Could you check a few things on this model? Use its own coordinates, in mm. A direction names the side the tool comes from. Give positions to 0.01 mm unless a question says otherwise; leave off trailing zeros. Loops run counter-clockwise (first coordinate to the right, second up) from the corner with the lowest first, then second, coordinate; pieces in that order, holes last. Notation, with made-up numbers: M -5,-35 L 17,-35 A20 cw 17,-9 Z; hole C 36,-36.5 d8. An arc over 180 degrees is marked long. Use CSV: the item, a comma, the result in double quotes.
```python
from build123d import *

# Parameters (mm, degrees)
BOSS_EXTRUDE1_DEPTH = 50
SKETCH2_W           = 7
SKETCH2_H           = 8
BOSS_EXTRUDE2_DEPTH = 50
SKETCH2_3_W         = 7
SKETCH2_3_H         = 8
BOSS_EXTRUDE3_DEPTH = 18
SKETCH3_W           = 10
SKETCH3_H           = 63
SKETCH3_W_2         = 7
SKETCH3_H_2         = 8
BOSS_EXTRUDE4_DEPTH = 82
FILLET1_R           = 5
SKETCH4_W           = 49
SKETCH4_H           = 29.5
CUT_EXTRUDE1_DEPTH  = 63
SKETCH5_W           = 29.5
SKETCH5_H           = 11
BOSS_EXTRUDE5_DEPTH = 49
CUT_EXTRUDE2_DEPTH  = 29.5
SKETCH6_R           = 1.75
CUT_EXTRUDE3_DEPTH  = 5
SKETCH6_6_R         = 0.75
CUT_EXTRUDE4_DEPTH  = 15
SKETCH8_W           = 18
SKETCH8_H           = 9.5
CUT_EXTRUDE5_DEPTH  = 40
SKETCH9_W           = 7
SKETCH9_H           = 9.5
CUT_EXTRUDE6_DEPTH  = 45
SKETCH10_W          = 10
SKETCH10_H          = 10
CUT_EXTRUDE7_DEPTH  = 29.5
SKETCH11_W          = 13
SKETCH11_H          = 48
SKETCH11_H_2        = 7
CUT_EXTRUDE8_DEPTH  = 124.13610356
SKETCH12_W          = 8
SKETCH12_H          = 10
CUT_EXTRUDE9_DEPTH  = 114.279521539
SKETCH13_W          = 10
SKETCH13_H          = 6
CUT_EXTRUDE10_DEPTH = 14
SKETCH15_W          = 14
SKETCH15_H          = 6
CUT_EXTRUDE11_DEPTH = 128.218316291
FILLET2_R           = 3
SKETCH17_W          = 49
SKETCH17_H          = 62
BOSS_EXTRUDE6_DEPTH = 46.5
CUT_EXTRUDE12_START = -30
SKETCH18_W          = 45
SKETCH18_H          = 63
CUT_EXTRUDE12_DEPTH = 30
SKETCH19_W          = 45
SKETCH19_H          = 4
SKETCH19_H_2        = 27.35
BOSS_EXTRUDE7_DEPTH = 30
BOSS_EXTRUDE8_DEPTH = 3
SKETCH24_W          = 14
SKETCH24_H          = 10
CUT_EXTRUDE15_DEPTH = 112.778799421
SKETCH26_W          = 42
SKETCH26_H          = 31.65
CUT_EXTRUDE16_DEPTH = 8
SKETCH27_W          = 42
SKETCH27_H          = 38
CUT_EXTRUDE17_DEPTH = 7
SKETCH28_W          = 42
SKETCH28_H          = 38
CUT_EXTRUDE18_DEPTH = 7
SKETCH29_W          = 38
SKETCH29_H          = 45.65
CUT_EXTRUDE19_DEPTH = 7
SKETCH30_W          = 46.5
SKETCH30_H          = 6
CUT_EXTRUDE20_DEPTH = 131.599578866
CUT_EXTRUDE21_DEPTH = 127.610623567
SKETCH32_3_R        = 0.9
SKETCH32_3_R_2      = 0.75
CUT_EXTRUDE22_DEPTH = 6


with BuildPart() as part:
    # Sketch1 → Boss-Extrude1 (new body)
    with BuildSketch(Plane.XY):
        with BuildLine():
            Line((-2.25, -8), (-4.25, -8))
            ThreePointArc((-4.25, -8), (-3.25, -8.5), (-2.25, -8))
        make_face()
        Polygon((10, -25.5), (10, 0), (0, 0), (-18, 0), (-18, -8), (0, -8), (0, -17.5), (-18, -17.5), (-18, -25.5), align=None)
    extrude(amount=BOSS_EXTRUDE1_DEPTH)

    # Sketch2 → Boss-Extrude2 (add)
    with BuildSketch(Plane(origin=(0, 0, 0), x_dir=(0, 0, -1), z_dir=(1, 0, 0))):
        Polygon((7, 0), (0, 0), (0, -8), (2.25, -8), (4.25, -8), (7, -8), align=None)
        Polygon((0, -8), (0, 0), (-10, 0), (-10, -25.5), (0, -25.5), (0, -17.5), align=None)
        with Locations((3.5, -21.5)):
            Rectangle(SKETCH2_W, SKETCH2_H)
        with BuildLine():
            Line((4.25, -8), (2.25, -8))
            ThreePointArc((2.25, -8), (3.25, -8.5), (4.25, -8))
        make_face()
    extrude(amount=BOSS_EXTRUDE2_DEPTH)

    # Sketch2<3> → Boss-Extrude3 (add)
    with BuildSketch(Plane(origin=(0, 0, 0), x_dir=(0, 0, -1), z_dir=(1, 0, 0))):
        Polygon((7, 0), (0, 0), (0, -8), (2.25, -8), (4.25, -8), (7, -8), align=None)
        with Locations((3.5, -21.5)):
            Rectangle(SKETCH2_3_W, SKETCH2_3_H)
    extrude(amount=-BOSS_EXTRUDE3_DEPTH)

    # Sketch3 → Boss-Extrude4 (add)
    with BuildSketch(Plane(origin=(50, 0, 0), x_dir=(0, 0, -1), z_dir=(1, 0, 0))):
        Polygon((36.5, -17.5), (7, -17.5), (7, -25.5), (0, -25.5), (0, -88.5), (36.5, -88.5), align=None)
        with Locations((-5, -57)):
            Rectangle(SKETCH3_W, SKETCH3_H)
        with Locations((3.5, -21.5)):
            Rectangle(SKETCH3_W_2, SKETCH3_H_2)
        with Locations((-5, -21.5)):
            Rectangle(SKETCH3_W, SKETCH3_H_2)
    extrude(amount=-BOSS_EXTRUDE4_DEPTH)

    # Fillet1
    fillet1_edges = [part.edges().sort_by_distance(p)[0] for p in [
        (-32, -17.5, -13.25),
        (-32, -53, -36.5),
        (9, -17.5, -36.5),
    ]]
    fillet(fillet1_edges, radius=FILLET1_R)

    # Sketch4 → Cut-Extrude1 (cut)
    with BuildSketch(Plane.XZ.offset(88.5)):
        with Locations((25.5, -4.75)):
            Rectangle(SKETCH4_W, SKETCH4_H)
    extrude(amount=-CUT_EXTRUDE1_DEPTH, mode=Mode.SUBTRACT)

    # Sketch5 → Boss-Extrude5 (add)
    with BuildSketch(Plane(origin=(50, 0, 0), x_dir=(0, 0, -1), z_dir=(1, 0, 0))):
        with Locations((4.75, -31)):
            Rectangle(SKETCH5_W, SKETCH5_H)
        with Locations((4.75, -83)):
            Rectangle(SKETCH5_W, SKETCH5_H)
    extrude(amount=-BOSS_EXTRUDE5_DEPTH)

    # Sketch7 → Cut-Extrude2 (cut)
    with BuildSketch(Plane.XY.offset(10)):
        Polygon((1, -36.5), (27, -36.5), (27, -26.5), (50, -26.5), (50, -88.5), (27, -88.5), (27, -77.5), (1, -77.5), align=None)
    extrude(amount=-CUT_EXTRUDE2_DEPTH, mode=Mode.SUBTRACT)

    # Sketch6 → Cut-Extrude3 (cut)
    with BuildSketch(Plane(origin=(27, 0, 0), x_dir=(0, 0, -1), z_dir=(1, 0, 0))):
        with Locations((4.25, -81.5)):
            Circle(SKETCH6_R)
        with Locations((14.25, -81.5)):
            Circle(SKETCH6_R)
        with Locations((14.25, -32.5)):
            Circle(SKETCH6_R)
        with Locations((4.25, -32.5)):
            Circle(SKETCH6_R)
    extrude(amount=-CUT_EXTRUDE3_DEPTH, mode=Mode.SUBTRACT)

    # Sketch6<6> → Cut-Extrude4 (cut)
    with BuildSketch(Plane(origin=(27, 0, 0), x_dir=(0, 0, -1), z_dir=(1, 0, 0))):
        with Locations((4.25, -81.5)):
            Circle(SKETCH6_6_R)
        with Locations((14.25, -81.5)):
            Circle(SKETCH6_6_R)
        with Locations((14.25, -32.5)):
            Circle(SKETCH6_6_R)
        with Locations((4.25, -32.5)):
            Circle(SKETCH6_6_R)
    extrude(amount=-CUT_EXTRUDE4_DEPTH, mode=Mode.SUBTRACT)

    # Sketch8 → Cut-Extrude5 (cut)
    with BuildSketch(Plane(origin=(0, 0, -7), x_dir=(-1, 0, 0), z_dir=(0, 0, -1))):
        with Locations((9, -12.75)):
            Rectangle(SKETCH8_W, SKETCH8_H)
    extrude(amount=-CUT_EXTRUDE5_DEPTH, mode=Mode.SUBTRACT)

    # Sketch9 → Cut-Extrude6 (cut)
    with BuildSketch(Plane.ZY.offset(18)):
        with Locations((-3.5, -12.75)):
            Rectangle(SKETCH9_W, SKETCH9_H)
    extrude(amount=-CUT_EXTRUDE6_DEPTH, mode=Mode.SUBTRACT)

    # Sketch10 → Cut-Extrude7 (cut)
    with BuildSketch(Plane.XY.offset(10)):
        with Locations((6, -31.5)):
            Rectangle(SKETCH10_W, SKETCH10_H)
    extrude(amount=-CUT_EXTRUDE7_DEPTH, mode=Mode.SUBTRACT)

    # Sketch11 → Cut-Extrude8 (cut, through all)
    with BuildSketch(Plane.XY.offset(-19.5)):
        with Locations((43.5, -57.5)):
            Rectangle(SKETCH11_W, SKETCH11_H)
        with Locations((43.5, -85)):
            Rectangle(SKETCH11_W, SKETCH11_H_2)
    extrude(amount=-CUT_EXTRUDE8_DEPTH, mode=Mode.SUBTRACT)

    # Sketch12 → Cut-Extrude9 (cut, through all)
    with BuildSketch(Plane.XZ.offset(88.5)):
        with Locations((-28, -31.5)):
            Rectangle(SKETCH12_W, SKETCH12_H)
    extrude(amount=-CUT_EXTRUDE9_DEPTH, mode=Mode.SUBTRACT)

    # Sketch13 → Cut-Extrude10 (cut)
    with BuildSketch(Plane.ZY.offset(32)):
        with Locations((-31.5, -20.5)):
            Rectangle(SKETCH13_W, SKETCH13_H)
    extrude(amount=-CUT_EXTRUDE10_DEPTH, mode=Mode.SUBTRACT)

    # Sketch15 → Cut-Extrude11 (cut, through all)
    with BuildSketch(Plane(origin=(0, 0, -26.5), x_dir=(-1, 0, 0), z_dir=(0, 0, -1))):
        with Locations((25, -20.5)):
            Rectangle(SKETCH15_W, SKETCH15_H)
    extrude(amount=-CUT_EXTRUDE11_DEPTH, mode=Mode.SUBTRACT)

    # Fillet2
    fillet2_edges = [part.edges().sort_by_distance(p)[0] for p in [
        (-24, -56, -26.5),
        (-24, -23.5, -31.5),
        (-28, -23.5, -26.5),
    ]]
    fillet(fillet2_edges, radius=FILLET2_R)

    # Sketch17 → Boss-Extrude6 (add)
    with BuildSketch(Plane.XY.offset(10)):
        with Locations((25.5, -57.5)):
            Rectangle(SKETCH17_W, SKETCH17_H)
    extrude(amount=-BOSS_EXTRUDE6_DEPTH)

    # Sketch18 → Cut-Extrude12 (cut)
    with BuildSketch(Plane.XY.offset(10).offset(CUT_EXTRUDE12_START)):
        with Locations((27.5, -57)):
            Rectangle(SKETCH18_W, SKETCH18_H)
    extrude(amount=CUT_EXTRUDE12_DEPTH, mode=Mode.SUBTRACT)

    # Sketch19 → Boss-Extrude7 (add)
    with BuildSketch(Plane.XY.offset(-20)):
        with Locations((27.5, -27.5)):
            Rectangle(SKETCH19_W, SKETCH19_H)
        with Locations((27.5, -74.825)):
            Rectangle(SKETCH19_W, SKETCH19_H_2)
    extrude(amount=BOSS_EXTRUDE7_DEPTH)

    # Sketch22 → Boss-Extrude8 (add)
    with BuildSketch(Plane(origin=(50, 0, 0), x_dir=(0, 0, -1), z_dir=(1, 0, 0))):
        with BuildLine():
            Line((20, -61.15), (20, -45.325))
            Line((20, -45.325), (13.5, -45.325))
            ThreePointArc((13.5, -45.325), (11.01040764, -51.33540764), (5, -53.825))
            Line((5, -53.825), (5, -61.15))
            Line((5, -61.15), (20, -61.15))
        make_face()
        with BuildLine():
            Line((20, -45.325), (20, -29.5))
            Line((20, -29.5), (5, -29.5))
            Line((5, -29.5), (5, -36.825))
            ThreePointArc((5, -36.825), (11.01040764, -39.31459236), (13.5, -45.325))
            Line((13.5, -45.325), (20, -45.325))
        make_face()
    extrude(amount=-BOSS_EXTRUDE8_DEPTH)

    # Sketch24 → Cut-Extrude15 (cut, through all)
    with BuildSketch(Plane.XY.offset(10)):
        with Locations((-25, -28.5)):
            Rectangle(SKETCH24_W, SKETCH24_H)
    extrude(amount=-CUT_EXTRUDE15_DEPTH, mode=Mode.SUBTRACT)

    # Sketch26 → Cut-Extrude16 (cut)
    with BuildSketch(Plane.XY.offset(-20)):
        with Locations((26, -45.325)):
            Rectangle(SKETCH26_W, SKETCH26_H)
    extrude(amount=-CUT_EXTRUDE16_DEPTH, mode=Mode.SUBTRACT)

    # Sketch27 → Cut-Extrude17 (cut)
    with BuildSketch(Plane.XZ.offset(29.5)):
        with Locations((26, -9)):
            Rectangle(SKETCH27_W, SKETCH27_H)
    extrude(amount=-CUT_EXTRUDE17_DEPTH, mode=Mode.SUBTRACT)

    # Sketch28 → Cut-Extrude18 (cut)
    with BuildSketch(Plane(origin=(0, -61.15, 0), x_dir=(1, 0, 0), z_dir=(0, 1, 0))):
        with Locations((26, 9)):
            Rectangle(SKETCH28_W, SKETCH28_H)
    extrude(amount=-CUT_EXTRUDE18_DEPTH, mode=Mode.SUBTRACT)

    # Sketch29 → Cut-Extrude19 (cut)
    with BuildSketch(Plane(origin=(5, 0, 0), x_dir=(0, 0, -1), z_dir=(1, 0, 0))):
        with Locations((9, -45.325)):
            Rectangle(SKETCH29_W, SKETCH29_H)
    extrude(amount=-CUT_EXTRUDE19_DEPTH, mode=Mode.SUBTRACT)

    # Sketch30 → Cut-Extrude20 (cut, through all)
    with BuildSketch(Plane(origin=(50, 0, 0), x_dir=(0, 0, -1), z_dir=(1, 0, 0))):
        with Locations((13.25, -85.5)):
            Rectangle(SKETCH30_W, SKETCH30_H)
    extrude(amount=-CUT_EXTRUDE20_DEPTH, mode=Mode.SUBTRACT)

    # Sketch32 → Cut-Extrude21 (cut, through all)
    with BuildSketch(Plane(origin=(50, 0, 0), x_dir=(0, 0, -1), z_dir=(1, 0, 0))):
        with BuildLine():
            ThreePointArc((36.5, -22.5), (35.035533906, -18.964466094), (31.5, -17.5))
            Line((31.5, -17.5), (29.5, -17.5))
            Line((29.5, -17.5), (29.5, -20))
            Line((29.5, -20), (29.5, -21))
            Line((29.5, -21), (29.5, -24.5))
            Line((29.5, -24.5), (33, -24.5))
            Line((33, -24.5), (34.1, -24.5))
            Line((34.1, -24.5), (35.4, -24.5))
            Line((35.4, -24.5), (36.5, -24.5))
            Line((36.5, -24.5), (36.5, -22.5))
        make_face()
    extrude(amount=-CUT_EXTRUDE21_DEPTH, mode=Mode.SUBTRACT)

    # Sketch32<3> → Cut-Extrude22 (cut)
    with BuildSketch(Plane(origin=(50, 0, 0), x_dir=(0, 0, -1), z_dir=(1, 0, 0))):
        with Locations((27.75, -22.75)):
            Circle(SKETCH32_3_R)
        with Locations((27.75, -22.75)):
            Circle(SKETCH32_3_R_2, mode=Mode.SUBTRACT)
        with Locations((27.75, -22.75)):
            Circle(SKETCH32_3_R_2)
        with Locations((31.25, -26.25)):
            Circle(SKETCH32_3_R)
        with Locations((31.25, -26.25)):
            Circle(SKETCH32_3_R_2, mode=Mode.SUBTRACT)
        with Locations((31.25, -26.25)):
            Circle(SKETCH32_3_R_2)
    extrude(amount=-CUT_EXTRUDE22_DEPTH, mode=Mode.SUBTRACT)


solid = part.part
```
1. I want a section at B-B, the plane x = 34. List the corners of the cut face in (y, z) for me.
Outcome:
outline,"M -82.5,-36.5 L -24.5,-36.5 L -24.5,-29.5 L -17.5,-29.5 L -17.5,0 L -8,0 L -8,-2.25 A1.25 ccw -8,-4.25 L -8,-7 L 0,-7 L 0,10 L -22.5,10 L -22.5,-28 L -68.15,-28 L -68.15,10 L -82.5,10 Z"
2. Please list where these lines run through material, in increasing order: line 1 (Y direction, x = 48.25, z = -27.75); line 2 (Y direction, x = 32.5, z = -26.5); line 3 (X direction, y = -68, z = -4.5).
Outcome:
line 1,"-82.5 to -23.65, -21.85 to -17.5"
line 2,"-82.5 to -68.15, -22.5 to -17.5"
line 3,"-32 to -2, 47 to 50"
3. I'm going to push flat-ended pins straight in: pin 1 Ø3.5 at (x, y) = (14.5, -19.5) entering from -Z; pin 2 Ø3 at (x, z) = (20, -25.5) entering from +Y; pin 3 Ø2 at (y, z) = (-11, 16.5) entering from -X. Where does each tip first touch, or does it pass through?
Outcome:
pin 1,"z = -29.5"
pin 2,"y = -17.5"
pin 3,"x = 0"
4. I want a section at D-D, the plane y = -11.5. List the corners of the cut face in (x, z) for me.
Outcome:
outline,"M 0,0 L 50,0 L 50,10 L 10,10 L 10,50 L 0,50 Z"
5. I want a section at A-A, the plane z = -20. List the corners of the cut face in (x, y) for me.
Outcome:
outline,"M -32,-82.5 L 50,-82.5 L 50,-17.5 L -18,-17.5 L -18,-33.5 L -32,-33.5 Z; hole M -2,-68.15 L 47,-68.15 L 47,-22.5 L -2,-22.5 Z"
6. If we mould it in two halves opening along X, with no side actions, what happens to faces 4 (the face through (-10, -60, 10)), 5 (the face through (4, -24, 10)), 6 (the face through (-32, -58, -8))? For each: +X half, -X half, draft (parallel to the pull), parting line (faces both ways), or undercut.
Outcome:
face 4,"draft"
face 5,"undercut"
face 6,"-X half"
7. I want a section at C-C, the plane z = 24. List the corners of the cut face in (x, y) for me, then the cut area to 3 significant figures.
Outcome:
outline,"M -18,-25.5 L 10,-25.5 L 10,0 L -18,0 L -18,-8 L 0,-8 L 0,-17.5 L -18,-17.5 Z"
area,"543 mm2"
8. Which directions (+Z, -Z, +X, -X, +Y, -Y) give clear straight access to the entire face, cutting with the end or side of a thin tool? Please do faces 1 (the face through (-4, -25.5, 30)), 2 (the face through (22, -22.5, -9)), 3 (the face through (-18, -24, -2)).
Outcome:
face 1,"+Z, +X, -X, -Y"
face 2,"none"
face 3,"+Z, -Z, -X, +Y"
